from build123d import *

# Parameters (mm, degrees)
SKETCH1_W               = 50
SKETCH1_H               = 70
BOSS_EXTRUDE1_DEPTH     = 2
SKETCH2_R               = 5
SKETCH2_R_2             = 2.5
BOSS_EXTRUDE2_DEPTH     = 70
SKETCH3_R               = 2.5
CUT_EXTRUDE1_DEPTH      = 47.786750261
CUT_EXTRUDE2_DEPTH      = 47.786750261
CUT_EXTRUDE2_DEPTH_BACK = 47.786750261
SKETCH5_W               = 10
SKETCH5_H               = 14


with BuildPart() as part:
    # Sketch1 → Boss-Extrude1 (new body)
    with BuildSketch(Plane(origin=(0, 0, 0), x_dir=(1, 0, 0), z_dir=(0, 1, 0))):
        Rectangle(SKETCH1_W, SKETCH1_H)
    extrude(amount=BOSS_EXTRUDE1_DEPTH)

    # Sketch2 → Boss-Extrude2 (add)
    with BuildSketch(Plane.XY.offset(35)):
        with Locations((-25, 5)):
            Circle(SKETCH2_R)
        with Locations((-25, 5)):
            Circle(SKETCH2_R_2, mode=Mode.SUBTRACT)
    extrude(amount=-BOSS_EXTRUDE2_DEPTH)

    # Sketch3 → Cut-Extrude1 (cut, through all)
    with BuildSketch(Plane(origin=(0, 2, 0), x_dir=(1, 0, 0), z_dir=(0, 1, 0))):
        with Locations(Location((0, 15, 0), (0, 0, 270))):
            Circle(SKETCH3_R)
        with Locations(Location((0, -15, 0), (0, 0, 270))):
            Circle(SKETCH3_R)
    extrude(amount=-CUT_EXTRUDE1_DEPTH, mode=Mode.SUBTRACT)

    # Sketch5 → Cut-Extrude2 (cut, two sides: drawn at the far end of the back side and taken through both)
    with BuildSketch(Plane(origin=(0, 2, 0), x_dir=(1, 0, 0), z_dir=(0, 1, 0)).offset(-CUT_EXTRUDE2_DEPTH_BACK)):
        with Locations((-25, -14)):
            Rectangle(SKETCH5_W, SKETCH5_H)
        with Locations((-25, 14)):
            Rectangle(SKETCH5_W, SKETCH5_H)
    extrude(amount=CUT_EXTRUDE2_DEPTH + CUT_EXTRUDE2_DEPTH_BACK, mode=Mode.SUBTRACT)


solid = part.part
The model under review builds one solid part; all positions refer to its coordinate system, in mm. A direction names the side the tool comes from. Give positions to 0.01 mm unless a question says otherwise; leave off trailing zeros. Write each loop counter-clockwise with the first axis right and the second up, starting at its lowest first coordinate (ties: lowest second). Pieces come first, ordered by that corner, then holes.
1. Draft analysis for pull direction Z (two halves, no side actions). For faces 1 (the flat face through (-11, 1, 35)), 2 (the cylindrical face through (-26.84, 6.69, -27.9)), 3 (the flat face through (-20, 1, -14)), 4 (the flat face through (-23, 3, -21)), state which applies: +Z half, -Z half, draft (parallel to the pull), parting line (faces both ways), or undercut.
2. Add section C-C, the plane x = -18. Write out the cut boundary in (y, z), plus the area to 3 significant figures.
3. Tool access review of faces 5 (the cylindrical face through (-26.84, 6.69, 0.1)), 6 (the flat face through (-23, 3, 7)): name each direction out of +Z, -Z, +X, -X, +Y, -Y from which nothing blocks a thin tool from reaching the whole face with its end or side.
4. Add section B-B, the plane z = -6. Write out the cut boundary in (x, y).
5. For P1, Ø6, axis at x = -19.5, y = 9, coming from the -Z side; P2, Ø1.6, axis at y = 1.5, z = -11.5, coming from the -X side; P3, Ø6.5, axis at x = 0, z = 15, coming from the +Y side; P4, Ø3, axis at y = 7.5, z = 22, coming from the +X side, all flat-tipped, find the tip position at first contact; note any pin that passes through.
6. Add section A-A, the plane z = 15. Write out the cut boundary in (x, y).
7. Wall thickness on L1, parallel to Z at x = -21, y = 7.25; L2, parallel to X at y = 0.6, z = -15; L3, parallel to Y at x = -25, z = -1: over which ranges is each line inside the solid? List them lowest first.
Worked answers:
1. face 1: +Z half
1. face 2: draft
1. face 3: undercut
1. face 4: undercut
2. outline: (0, -35) - (2, -35) - (2, 35) - (0, 35) - close
2. area: 140 mm2
3. face 5: +Z, -Z
3. face 6: -X, +Y, -Y
4. outline: (-25, 0) - (25, 0) - (25, 2) - (-21, 2) arc R5 ccw (long way) to start; hole circle Ø5 at (-25, 5)
5. P1: stops at z = -35
5. P2: stops at x = -20
5. P3: stops at y = 2
5. P4: stops at x = -20.1
6. outline: (-20, 0) - (-2.5, 0) - (-2.5, 2) - (-20, 2) - close; (2.5, 0) - (25, 0) - (25, 2) - (2.5, 2) - close
7. L1: z = -35 to -21, -7 to 7, 21 to 35
7. L2: x = -20 to -2.5, 2.5 to 25
7. L3: y = 0 to 2.5, 7.5 to 10
